Verification items for the finished model (mm, model axes). A direction names the side the tool comes from. Give positions to 0.01 mm unless a question says otherwise; leave off trailing zeros. Write each loop counter-clockwise with the first axis right and the second up, starting at its lowest first coordinate (ties: lowest second). Pieces come first, ordered by that corner, then holes. Notation, with made-up numbers: (16.5, 7.5) -> (65.5, 7.5) arc R21 cw to (65.5, 45.5) -> close; hole circle Ø5 at (-11, 71). An arc over 180 degrees is marked (long way). Use one line per item in the form item = value. Start each with the question number.
(1) Section check B-B, the plane y = -3.5. Record the cut outline in (x, z), plus the area to 3 significant figures.
(2) Set-up check for faces 1 (the face through (5.95, -4, -16)), 2 (the face through (-2.25, 0, -10)), 3 (the face through (-5.95, 0, -6)): record each of +Z, -Z, +X, -X, +Y, -Y from which the full face is reachable in a straight line by a thin tool's end or side.
(3) Release check for a two-part mould opening along X. For faces 4 (the face through (5.95, 0, -6)), 5 (the face through (-7.45, -2, -16)), 6 (the face through (-0.032, 0.724, -2.738)) record: pulls with the +X half, pulls with the -X half, needs draft (parallel to the pull), parting line crosses it, or undercut.
(4) Scan lines: L1, parallel to X at y = 0, z = -16.15; L2, parallel to Z at x = -1.25, y = -1.75; L3, parallel to Y at x = 0, z = -16.85. Record each from-to range of solid material in increasing order.
(5) Section check D-D, the plane z = -15.25. Record the cut outline in (x, y).
(6) Section check A-A, the plane z = -5.75. Record the cut outline in (x, y), plus the area to 3 significant figures.
(7) Section check C-C, the plane x = 0. Record the cut outline in (y, z) (3 decimals), plus the area to 3 significant figures.
(8) Depth check by flat-ended pin: pin 1 Ø2 at (y, z) = (1, -4) entering from +X; pin 2 Ø8 at (x, z) = (2, -12.5) entering from -Y; pin 3 Ø0.8 at (x, y) = (-6.5, -4.5) entering from +Z. Enter the tip coordinate at first touch or a pass-through.
Autodesk Inventor part; units mm, degrees
ref_plane "YZ Plane" through (0, 0, 0) normal (1, 0, 0) x (0, 1, 0)
ref_plane "XZ Plane" through (0, 0, 0) normal (0, 1, 0) x (-1, 0, 0)
ref_plane "XY Plane" through (0, 0, 0) normal (0, 0, 1) x (1, 0, 0)
sketch "Sketch6" plane through (0, 0, 0) normal (0, 0, 1) x (1, 0, 0)
  line L0 (-5.95, 2.3) -> (5.95, 2.3)
  line L1 (5.95, 2.3) -> (5.95, -2.3)
  line L2 (5.95, -2.3) -> (-5.95, -2.3)
  line L3 (-5.95, -2.3) -> (-5.95, 2.3)
  line L4 (-5.95, 2.3) -> (5.95, -2.3) construction
  line L5 (5.95, 2.3) -> (-5.95, -2.3) construction
  point P0 (0, 0)
  point P1 (0, 0)
  dimension "d66" = 11.9
  dimension "d67" = 4.6
extrude "Extrusion6" add sketch "Sketch6" against normal blind 18.4
hole "Hole6" at (0, 0, 0) direction (0, 0, -1) diameter 1.45 depth 7 tip angle 118
sketch "Sketch7" plane through (5.95, -2.3, 0) normal (1, 0, 0) x (0, 0, -1)
  line L0 (18.4, 4.6) -> (13.7908, 4.6)
  line L1 (13.7908, 4.6) -> (13.7908, -3.6343)
  line L2 (13.7908, -3.6343) -> (18.4, -3.6343)
  line L3 (18.4, -3.6343) -> (18.4, 4.6)
  point P0 (0, 2.3)
extrude "Extrusion7" add sketch "Sketch7" along normal blind 1.5
ref_plane "Work Plane13" through (0, -2.3, 0) normal (1, 0, 0) x (0, 0, -1)
mirror "Mirror1" about plane through (0, -2.3, 0) normal (1, 0, 0) of "Extrusion7"
fillet "Fillet3" radius 2 2 edges at (5.95, 0, -13.7908) (-5.95, 0, -13.7908)
sketch "Sketch8" plane through (-5.95, 2.3, 0) normal (0, 1, 0) x (1, 0, 0)
  line L0 (3.7, 5.4) -> (8.2, 5.4)
  line L1 (8.2, 5.4) -> (8.2, 14.4)
  line L2 (8.2, 14.4) -> (3.7, 14.4)
  line L3 (3.7, 14.4) -> (3.7, 5.4)
  line L4 (3.7, 5.4) -> (8.2, 14.4) construction
  line L5 (8.2, 5.4) -> (3.7, 14.4) construction
  line L6 (5.95, 22.08) -> (5.95, -3.68) construction
  line L7 (13.4, 18.4) -> (-1.5, 18.4)
  point P0 (5.95, 0)
  point P1 (5.95, 9.9)
  point P2 (5.95, 9.9)
  dimension "d87" = 4
  dimension "d88" = 4.5
  dimension "d101" = 9
extrude "Extrusion8" cut sketch "Sketch8" against normal through all
ref_plane "Work Plane14" through (-5.95, 0, 0) normal (0, 1, 0) x (1, 0, 0)
hole "Hole7" at (0, 0, -18.4) direction (0, 0, 1) diameter 1.48 depth 7 tip angle 118
properties part number "servo_attachement" material "ABS Plastic"
Completed:
q1.outline = (-7.45, -18.4) -> (-5.95, -18.4) -> (-5.95, -13.79) -> (-7.45, -13.79) -> close; (5.95, -18.4) -> (7.45, -18.4) -> (7.45, -13.79) -> (5.95, -13.79) -> close
q1.area = 13.8 mm²
q2.face_1 = +Z, -Z, -Y
q2.face_2 = +Y, -Y
q2.face_3 = +Z, -X, +Y, -Y
q3.face_4 = pulls with the +X half
q3.face_5 = pulls with the -X half
q3.face_6 = undercut
q4.L1 = -7.45 to -0.74, 0.74 to 7.45
q4.L2 = -18.4 to -14.4, -5.4 to 0
q4.L3 = -2.3 to -0.74, 0.74 to 2.3
q5.outline = (-7.45, -5.93) -> (-5.95, -5.93) -> (-5.95, -2.3) -> (5.95, -2.3) -> (5.95, -5.93) -> (7.45, -5.93) -> (7.45, 2.3) -> (-7.45, 2.3) -> close; hole circle Ø1.48 at (0, 0)
q6.outline = (-5.95, -2.3) -> (-2.25, -2.3) -> (-2.25, 2.3) -> (-5.95, 2.3) -> close; (2.25, -2.3) -> (5.95, -2.3) -> (5.95, 2.3) -> (2.25, 2.3) -> close
q6.area = 34.0 mm²
q7.outline = (-2.3, -18.4) -> (-0.74, -18.4) -> (-0.74, -14.4) -> (-2.3, -14.4) -> close; (-2.3, -5.4) -> (-0.725, -5.4) -> (-0.725, 0) -> (-2.3, 0) -> close; (0.725, -5.4) -> (2.3, -5.4) -> (2.3, 0) -> (0.725, 0) -> close; (0.74, -18.4) -> (2.3, -18.4) -> (2.3, -14.4) -> (0.74, -14.4) -> close
q7.area = 29.5 mm²
q8.pin_1 = 5.95
q8.pin_2 = -2.3
q8.pin_3 = -13.79
